Verification items for this drawing (mm, ordinates from the low corner). A direction names the side the tool comes from. Coordinates: 2 decimals unless noted, no trailing zeros. Order: outer loops, then holes, each group sorted by start corner. A loop starts at its lowest first (then second) coordinate and runs counter-clockwise, first axis right, second up. Notation, with made-up numbers: (-8, -19.5) -> (24, -19.5) arc R22 cw to (24, -9.5) -> close; hole circle Ø11 at (-10.75, 50). An arc over 180 degrees is marked (long way). Write item = value, one per line. Start each with the question number.
1. Thickness scan on line 1 along Z through (x, y) = (42, 7.5); line 2 along X through (y, z) = (2.25, 7.5); line 3 along X through (y, z) = (2, 4.75). Record the ranges inside material, lowest first. Write a range as from..to.
2. Go/stop test with flat-tipped pins: P1, Ø5, axis at x = 42, z = 5, coming from the +Y side; P2, Ø1, axis at x = 5, y = 9, coming from the +Z side. Record where each tip stops, or that it passes through.
3. Cross-section at C-C on z = 7.75. Record the cut outline in (x, y).
4. Cross-section at D-D on x = 3. Record the cut outline in (y, z).
5. Release check for a two-part mould opening along X. For the marked faces 3, 4, 5 and 6 record: +X half, -X half, draft (parallel to the pull), parting line (faces both ways), or undercut.
6. Set-up check for the marked faces 1 and 2: record each of +Z, -Z, +X, -X, +Y, -Y from which the full face is reachable in a straight line by a thin tool's end or side.
7. Cross-section at B-B on x = 42. Record the cut outline in (y, z).
8. Cross-section at A-A on y = 3. Record the cut outline in (x, z), plus the area to 3 significant figures.
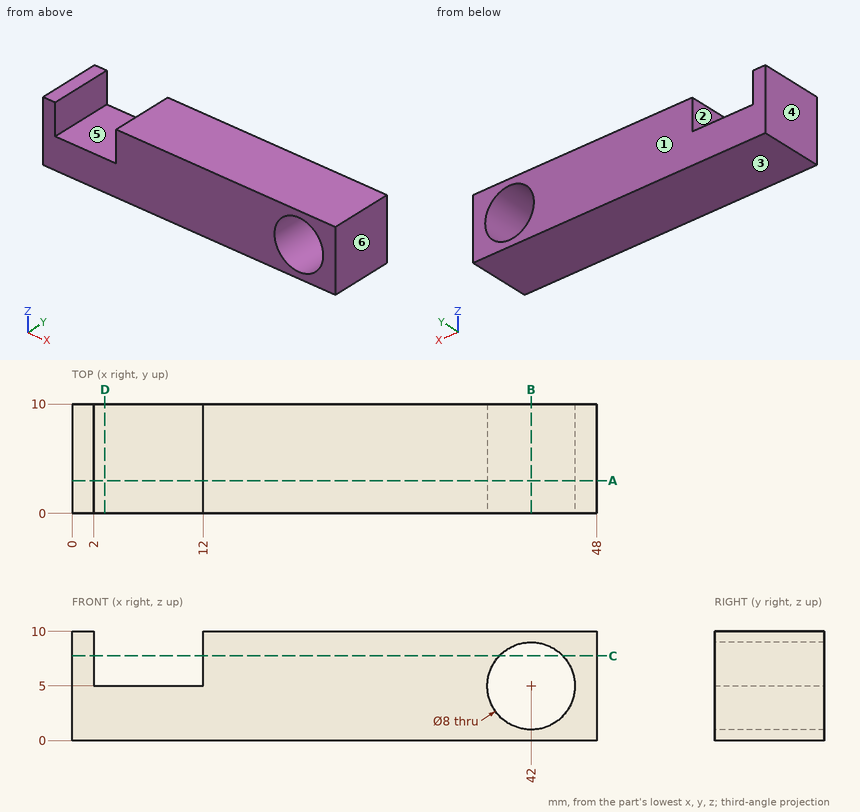
Worked out:
q1.line_1 = 0..1, 9..10
q1.line_2 = 0..2, 12..38.88, 45.12..48
q1.line_3 = 0..38.01, 45.99..48
q2.P1 = through
q2.P2 = 5
q3.outline = (0, 0) -> (2, 0) -> (2, 10) -> (0, 10) -> close; (12, 0) -> (39.1, 0) -> (39.1, 10) -> (12, 10) -> close; (44.9, 0) -> (48, 0) -> (48, 10) -> (44.9, 10) -> close
q4.outline = (0, 0) -> (10, 0) -> (10, 5) -> (0, 5) -> close
q5.face_3 = draft
q5.face_4 = -X half
q5.face_5 = undercut
q5.face_6 = +X half
q6.face_1 = +Z, -Z, +X, -X, +Y
q6.face_2 = +Z, +Y, -Y
q7.outline = (0, 0) -> (10, 0) -> (10, 1) -> (0, 1) -> close; (0, 9) -> (10, 9) -> (10, 10) -> (0, 10) -> close
q8.outline = (0, 0) -> (48, 0) -> (48, 10) -> (12, 10) -> (12, 5) -> (2, 5) -> (2, 10) -> (0, 10) -> close; hole circle Ø8 at (42, 5)
q8.area = 380 mm²
